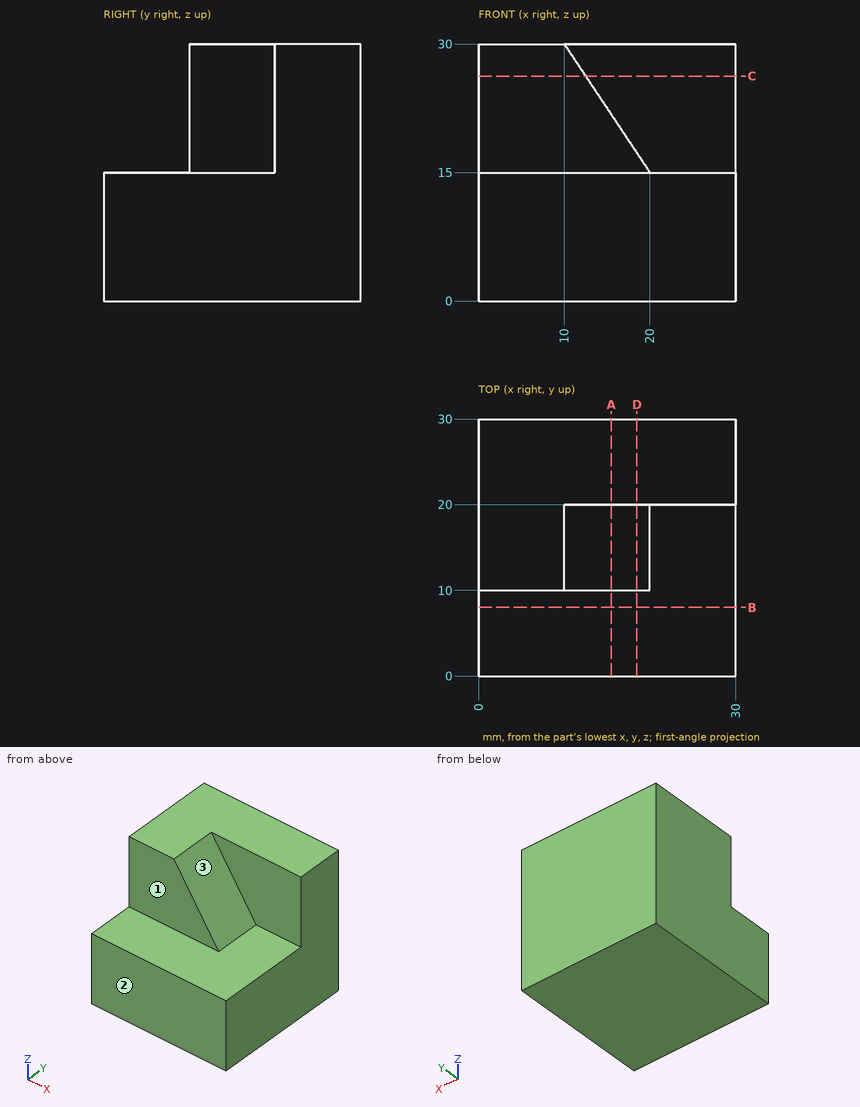
Design review of the part shown in the three views and the two pictorial views. Dimensions are in mm from the part's minimum x, y and z. A direction names the side the tool comes from. Coordinates: 2 decimals unless noted, no trailing zeros. Loops run counter-clockwise (first coordinate to the right, second up) from the corner with the lowest first, then second, coordinate; pieces in that order, holes last.
Q1. To check wall thickness, follow line 1 (Y direction, x = 25.5, z = 28.25); line 2 (Y direction, x = 7.25, z = 26); line 3 (Z direction, x = 21.75, y = 14.75). State the ranges of each line that lie inside material, in increasing order.
Reported:
line 1: y = 20 to 30
line 2: y = 10 to 30
line 3: z = 0 to 15
Q2. We need section D-D on x = 18.5. State the section outline as (y, z) points, and give its area (4 significant figures).
Reported:
outline: (0, 0) - (30, 0) - (30, 30) - (20, 30) - (20, 17.25) - (10, 17.25) - (10, 15) - (0, 15) - close
area: 622.5 mm2
Q3. We need section B-B on y = 8. State the section outline as (x, z) points, and give its area (3 significant figures).
Reported:
outline: (0, 0) - (30, 0) - (30, 15) - (0, 15) - close
area: 450 mm2
Q4. Tool access review of the marked faces 1, 2 and 3: name each direction out of +Z, -Z, +X, -X, +Y, -Y from which nothing blocks a thin tool from reaching the whole face with its end or side.
Reported:
face 1: +Z, +X, -X, -Y
face 2: +Z, -Z, +X, -X, -Y
face 3: +Z, +X, -Y
Q5. We need section C-C on z = 26.25. State the section outline as (x, y) points, and give its area (3 significant figures).
Reported:
outline: (0, 10) - (12.5, 10) - (12.5, 20) - (30, 20) - (30, 30) - (0, 30) - close
area: 425 mm2
Q6. For pin 1 (2 mm diameter, centred on x = 22.5, y = 6, fed in from +Z); pin 2 (16.5 mm diameter, centred on x = 9, z = 26, fed in from -Y), all flat-tipped, find the tip position at first contact; note any pin that passes through.
Reported:
pin 1: stops at z = 15
pin 2: stops at y = 10
Q7. We need section A-A on x = 15.5. State the section outline as (y, z) points.
Reported:
outline: (0, 0) - (30, 0) - (30, 30) - (20, 30) - (20, 21.75) - (10, 21.75) - (10, 15) - (0, 15) - close
